For this review, take the finished solid that the model builds, in its own axes (mm). A direction names the side the tool comes from. Coordinates: 2 decimals unless noted, no trailing zeros. Loops run counter-clockwise (first coordinate to the right, second up) from the corner with the lowest first, then second, coordinate; pieces in that order, holes last.
1. Take a section at D-D, the plane x = 9. State the section outline as (y, z) points, then the cut area to 3 significant figures.
2. Mouldability with a two-part tool opening along X and no side actions: class faces 1 (the face through (11.85, -0.41, -0.02)), 2 (the face through (0.2, -7.5, 0)), 3 (the face through (0, 22, 0)) as pulls with the +X half, pulls with the -X half, needs draft (parallel to the pull), parting line crosses it, or undercut.
3. Take a section at C-C, the plane y = 20. State the section outline as (x, z) points, then the cut area to 3 significant figures.
4. To check wall thickness, follow probe 1 along Y at (x, z) = (0, 0.3); probe 2 along X at (y, z) = (6.5, 1.05); probe 3 along X at (y, z) = (19, 0.4). State the ranges of each line that lie inside material, in increasing order.
5. Take a section at A-A, the plane x = 0. State the section outline as (y, z) points.
6. Machinability: for faces 4 (the face through (0, 9, 1.25)), 5 (the face through (9, 0, 0)), 6 (the face through (-9, 0, 0)), which of the approach directions +Z, -Z, +X, -X, +Y, -Y give a long, thin tool a straight path to every point of the face, cutting with its end or side? Answer none if there is none.
7. Take a section at B-B, the plane z = -0.5. State the section outline as (x, y) points.
8. Clearance check with flat-ended pins moving along their axes: P1, Ø0.8, axis at y = 6.5, z = -0.5, coming from the +X side; P2, Ø1.2, axis at y = 9.5, z = 0.5, coming from the -X side. State where each tip first meets the part, or that it passes through.
```python
from build123d import *

# Parameters (mm, degrees)
SKETCH1_R           = 2
BOSS_EXTRUDE1_DEPTH = 1.25
FILLET1_R           = 0.75


with BuildPart() as part:
    # Sketch1 → Boss-Extrude1 (new, symmetric)
    with BuildSketch(Plane.XY):
        with BuildLine():
            Line((7.75, 17.25), (7.75, 0))
            Line((7.75, 0), (12.5, 0))
            ThreePointArc((12.5, 0), (0, -7.5), (-12.5, 0))
            Line((-12.5, 0), (-7.75, 0))
            Line((-7.75, 0), (-7.75, 17.25))
            ThreePointArc((-7.75, 17.25), (0, 25), (7.75, 17.25))
        make_face()
        with Locations((0, 20)):
            Circle(SKETCH1_R, mode=Mode.SUBTRACT)
    extrude(amount=BOSS_EXTRUDE1_DEPTH, both=True)

    # Fillet1
    fillet1_edges = [part.edges().sort_by_distance(p)[0] for p in [
        (12.5, 0, 0),
        (-12.5, 0, 0),
    ]]
    fillet(fillet1_edges, radius=FILLET1_R)


solid = part.part
```
Results list:
1. outline: (-4.27, -1.25) - (0, -1.25) - (0, 1.25) - (-4.27, 1.25) - close
1. area: 10.7 mm2
2. face 1: pulls with the +X half
2. face 2: parting line crosses it
2. face 3: undercut
3. outline: (-7.25, -1.25) - (-2, -1.25) - (-2, 1.25) - (-7.25, 1.25) - close; (2, -1.25) - (7.25, -1.25) - (7.25, 1.25) - (2, 1.25) - close
3. area: 26.2 mm2
4. probe 1: y = -7.5 to 18, 22 to 25
4. probe 2: x = -7.75 to 7.75
4. probe 3: x = -7.55 to -1.73, 1.73 to 7.55
5. outline: (-7.5, -1.25) - (18, -1.25) - (18, 1.25) - (-7.5, 1.25) - close; (22, -1.25) - (25, -1.25) - (25, 1.25) - (22, 1.25) - close
6. face 4: +Z, +X, -X, +Y, -Y
6. face 5: +Z, -Z, +X, +Y
6. face 6: +Z, -Z, -X, +Y
7. outline: (-11.81, -1.16) arc R14.17 ccw to (11.81, -1.16) arc R0.75 ccw to (11.18, 0) - (7.75, 0) - (7.75, 17.25) arc R7.75 ccw to (-7.75, 17.25) - (-7.75, 0) - (-11.18, 0) arc R0.75 ccw to start; hole circle Ø4 at (0, 20)
8. P1: stops at x = 7.75
8. P2: stops at x = -7.75
